Work out the finished part from the listing and answer in its coordinate system (mm). A direction names the side the tool comes from. Round coordinates to 2 decimals unless told otherwise and drop trailing zeros. Order: outer loops, then holes, each group sorted by start corner. A loop starts at its lowest first (then second) coordinate and runs counter-clockwise, first axis right, second up. Notation, with made-up numbers: (70, -21.5) - (83, -21.5) arc R6 ccw to (83, -14.5) - close; hole circle Ø3 at (15.5, -34). An arc over 180 degrees is marked (long way). Put each result on its own line as item: value.
```python
from build123d import *

# Parameters (mm, degrees)
MODEL_R             = 1.5
MODEL_W             = 6
MODEL_H             = 2
BOSS_EXTRUDE1_DEPTH = 2


with BuildPart() as part:
    # Model → Boss-Extrude1 (new body)
    with BuildSketch(Plane.XY):
        with BuildLine():
            Line((1964.402734505, 1171.526635788), (1960.867200599, 1175.062169694))
            Line((1960.867200599, 1175.062169694), (1958.038773475, 1172.23374257))
            Line((1958.038773475, 1172.23374257), (1958.038773475, 1168.476383257))
            ThreePointArc((1958.038773475, 1168.476383257), (1958.917453131, 1166.355062913), (1961.038773475, 1165.476383257))
            Line((1961.038773475, 1165.476383257), (1963.867200599, 1165.476383257))
            Line((1963.867200599, 1165.476383257), (1964.195627724, 1165.476383257))
            ThreePointArc((1964.195627724, 1165.476383257), (1966.316948068, 1164.5977036), (1967.195627724, 1162.476383257))
            Line((1967.195627724, 1162.476383257), (1967.195627724, 1161.713700328))
            ThreePointArc((1967.195627724, 1161.713700328), (1968.074307381, 1159.592379984), (1970.195627724, 1158.713700328))
            Line((1970.195627724, 1158.713700328), (1979.195627724, 1158.713700328))
            ThreePointArc((1979.195627724, 1158.713700328), (1982.024054849, 1159.885273203), (1983.195627724, 1162.713700328))
            Line((1983.195627724, 1162.713700328), (1983.195627724, 1179.304810381))
            Line((1983.195627724, 1179.304810381), (1972.049181115, 1179.304810381))
            Line((1972.049181115, 1179.304810381), (1972.049181115, 1183.304810381))
            Line((1972.049181115, 1183.304810381), (1965.109841287, 1183.304810381))
            Line((1965.109841287, 1183.304810381), (1965.109841287, 1179.304810381))
            Line((1965.109841287, 1179.304810381), (1966.524054849, 1177.890596819))
            Line((1966.524054849, 1177.890596819), (1963.695627724, 1175.062169694))
            Line((1963.695627724, 1175.062169694), (1965.816948068, 1172.940849351))
            Line((1965.816948068, 1172.940849351), (1964.402734505, 1171.526635788))
        make_face()
        with Locations((1974.230460889, 1164.796116562)):
            Circle(MODEL_R, mode=Mode.SUBTRACT)
        with Locations((1976.195627724, 1176.304810381)):
            Rectangle(MODEL_W, MODEL_H, mode=Mode.SUBTRACT)
    extrude(amount=BOSS_EXTRUDE1_DEPTH)


solid = part.part
```
1) A cutting plane is placed at B-B on x = 1977. Write down the section's boundary in (y, z), then the cut area to 3 significant figures.
Findings below:
outline: (1158.71, 0) - (1175.3, 0) - (1175.3, 2) - (1158.71, 2) - close; (1177.3, 0) - (1179.3, 0) - (1179.3, 2) - (1177.3, 2) - close
area: 37.2 mm2
2) A cutting plane is placed at C-C on z = 1. Write down the section's boundary in (x, y), then the cut area to 3 significant figures.
Findings below:
outline: (1958.04, 1168.48) arc R3 ccw to (1961.04, 1165.48) - (1964.2, 1165.48) arc R3 cw to (1967.2, 1162.48) - (1967.2, 1161.71) arc R3 ccw to (1970.2, 1158.71) - (1979.2, 1158.71) arc R4 ccw to (1983.2, 1162.71) - (1983.2, 1179.3) - (1972.05, 1179.3) - (1972.05, 1183.3) - (1965.11, 1183.3) - (1965.11, 1179.3) - (1966.52, 1177.89) - (1963.7, 1175.06) - (1965.82, 1172.94) - (1964.4, 1171.53) - (1960.87, 1175.06) - (1958.04, 1172.23) - close; hole circle Ø3 at (1974.23, 1164.8); hole (1973.2, 1175.3) - (1979.2, 1175.3) - (1979.2, 1177.3) - (1973.2, 1177.3) - close
area: 416 mm2
3) A cutting plane is placed at D-D on y = 1180.25. Write down the section's boundary in (x, z).
Findings below:
outline: (1965.11, 0) - (1972.05, 0) - (1972.05, 2) - (1965.11, 2) - close
4) A cutting plane is placed at A-A on y = 1164.25. Write down the section's boundary in (x, z).
Findings below:
outline: (1966.62, 0) - (1972.83, 0) - (1972.83, 2) - (1966.62, 2) - close; (1975.63, 0) - (1983.2, 0) - (1983.2, 2) - (1975.63, 2) - close
5) Straight lines are drawn through the part: L1, parallel to Y at x = 1974.25, z = 0.9; L2, parallel to Y at x = 1976.25, z = 1.8; L3, parallel to Y at x = 1975, z = 0.75. For each, find the intervals that lie inside material, in ascending order. Write a range as from..to.
Findings below:
L1: y = 1158.71..1163.3, 1166.3..1175.3, 1177.3..1179.3
L2: y = 1158.71..1175.3, 1177.3..1179.3
L3: y = 1158.71..1163.51, 1166.08..1175.3, 1177.3..1179.3
6) For a pull along X with two mould halves and no side action, classify faces 4 (the flat face through (1958.039, 1170, 1)), 5 (the flat face through (1973, 1168, 0)), 6 (the flat face through (1962.66, 1173.27, 0.99)) as pulls with the +X half, pulls with the -X half, needs draft (parallel to the pull), parting line crosses it, or undercut.
Findings below:
face 4: pulls with the -X half
face 5: needs draft
face 6: undercut
7) For faces 1 (the flat face through (1965.11, 1181, 1)), 2 (the flat face through (1978, 1179.305, 1)), 3 (the flat face through (1965.12, 1172.244, 0.986)), determine the directions among +Z, -Z, +X, -X, +Y, -Y from which every point of the face is accessible in a straight line to the end or side of a thin tool.
Findings below:
face 1: +Z, -Z, -X, +Y
face 2: +Z, -Z, +X, +Y
face 3: +Z, -Z
8) Given pin 1 Ø0.8 at (y, z) = (1162, 1.5) entering from -X; pin 2 Ø1 at (x, z) = (1962, 1) entering from -Y; pin 3 Ø0.6 at (x, z) = (1979, 0.5) entering from +Y, each flat-ended and moving along its own axis, determine where each tip first touches the part or whether it passes through.
Findings below:
pin 1: stops at x = 1967.2
pin 2: stops at y = 1165.48
pin 3: stops at y = 1179.3
